Here's how the part is built. I have some questions about the finished solid (model axes, mm). A direction names the side the tool comes from. Round coordinates to 2 decimals unless told otherwise and drop trailing zeros. Order: outer loops, then holes, each group sorted by start corner. A loop starts at its lowest first (then second) coordinate and runs counter-clockwise, first axis right, second up. Notation, with made-up numbers: (-19, 78) -> (14, 78) arc R24 cw to (14, 102) -> close; hole circle Ø4 at (75, 84.5). An arc over 180 degrees is marked (long way). Answer in a Markdown table with one row per item.
```python
from build123d import *

# Parameters (mm, degrees)
SKETCH1_W           = 25
SKETCH1_H           = 50
SKETCH1_R           = 3.4
BOSS_EXTRUDE1_DEPTH = 3
SKETCH2_W           = 50
SKETCH2_H           = 3
BOSS_EXTRUDE2_DEPTH = 8
SKETCH3_W           = 8
SKETCH3_H           = 50
BOSS_EXTRUDE3_DEPTH = 42
SKETCH4_R           = 2.65
CUT_EXTRUDE1_DEPTH  = 0.5
SKETCH5_R           = 5.802370205
CUT_EXTRUDE2_DEPTH  = 9
FILLET2_R           = 1
SKETCH6_R           = 12.6
BOSS_EXTRUDE4_DEPTH = 2
FILLET4_R           = 1
SKETCH8_R           = 1.589780168
SKETCH8_R_2         = 1.777428262
CUT_EXTRUDE3_DEPTH  = 10
SKETCH9_W           = 49.021678163
SKETCH9_H           = 20.976854622
CUT_EXTRUDE4_DEPTH  = 68.79439129
SKETCH11_R          = 2.1
CUT_EXTRUDE5_DEPTH  = 59.480168703
SKETCH14_R          = 2.6
CUT_EXTRUDE6_DEPTH  = 0.5


with BuildPart() as part:
    # Sketch1 → Boss-Extrude1 (new body)
    with BuildSketch(Plane(origin=(0, 0, 0), x_dir=(1, 0, 0), z_dir=(0, 1, 0))):
        with Locations((2.276951673, 11.384758364)):
            Rectangle(SKETCH1_W, SKETCH1_H)
        with Locations(Location((1.276951673, 11.384758364, 0), (0, 0, 270))):
            Circle(SKETCH1_R, mode=Mode.SUBTRACT)
    extrude(amount=BOSS_EXTRUDE1_DEPTH)

    # Sketch2 → Boss-Extrude2 (add)
    with BuildSketch(Plane.ZY.offset(10.223048327)):
        with Locations((-11.384758364, 1.5)):
            Rectangle(SKETCH2_W, SKETCH2_H)
    extrude(amount=BOSS_EXTRUDE2_DEPTH)

    # Sketch3 → Boss-Extrude3 (add)
    with BuildSketch(Plane.XZ):
        with Locations((-14.223048327, -11.384758364)):
            Rectangle(SKETCH3_W, SKETCH3_H)
    extrude(amount=BOSS_EXTRUDE3_DEPTH)

    # Sketch4 → Cut-Extrude1 (cut)
    with BuildSketch(Plane(origin=(0, 3, 0), x_dir=(1, 0, 0), z_dir=(0, 1, 0))):
        with Locations(Location((-14.223048327, 32.384758364, 0), (0, 0, 270))):
            Circle(SKETCH4_R)
        with Locations(Location((-14.223048327, -9.615241636, 0), (0, 0, 270))):
            Circle(SKETCH4_R)
    cut_extrude1 = extrude(amount=-CUT_EXTRUDE1_DEPTH, mode=Mode.SUBTRACT)

    # Mirror1: Cut-Extrude1 across plane
    add(cut_extrude1.mirror(Plane.ZX.offset(-19.5)), mode=Mode.SUBTRACT)

    # Sketch5 → Cut-Extrude2 (cut)
    with BuildSketch(Plane.ZY.offset(18.223048327)):
        with Locations((-11.836279124, -21)):
            Circle(SKETCH5_R)
    extrude(amount=-CUT_EXTRUDE2_DEPTH, mode=Mode.SUBTRACT)

    # Fillet2
    fillet2_edges = [part.edges().sort_by_distance(p)[0] for p in [
        (-10.223048327, -21, -17.638649329),
    ]]
    fillet(fillet2_edges, radius=FILLET2_R)

    # Mirror2: Cut-Extrude1 across plane
    add(cut_extrude1.mirror(Plane.ZY.offset(1.723048327)), mode=Mode.SUBTRACT)

    # Sketch6 → Boss-Extrude4 (add)
    with BuildSketch(Plane(origin=(0, 3, 0), x_dir=(1, 0, 0), z_dir=(0, 1, 0))):
        with BuildLine():
            Line((14.776951673, 5.825082115), (14.776951673, 16.944434614))
            ThreePointArc((14.776951673, 16.944434614), (-13.323048327, 11.384758364), (14.776951673, 5.825082115))
        make_face()
        with Locations(Location((1.276951673, 11.384758364, 0), (0, 0, 270))):
            Circle(SKETCH6_R, mode=Mode.SUBTRACT)
    extrude(amount=BOSS_EXTRUDE4_DEPTH)

    # Fillet4
    # the kernel refuses this fillet: 1 mm, written as the material it takes off along each edge
    with BuildSketch(Plane(origin=(14.776951673, 5, -3.325082115), x_dir=(0, -1, 0), z_dir=(0, 0, -1))) as fillet4_piece_1:
        with BuildLine():
            CenterArc((FILLET4_R, FILLET4_R), FILLET4_R, 180, 90)
            Line((0, FILLET4_R), (0, 0))
            Line((0, 0), (FILLET4_R, 0))
        make_face()
    extrude(amount=16.119352499, mode=Mode.SUBTRACT)

    # Sketch8 → Cut-Extrude3 (cut)
    with BuildSketch(Plane(origin=(0, 3, 0), x_dir=(1, 0, 0), z_dir=(0, 1, 0))):
        with Locations(Location((1.276951673, 19.884758364, 0), (0, 0, 270))):
            Circle(SKETCH8_R)
        with Locations(Location((1.276951673, 2.884758364, 0), (0, 0, 270))):
            Circle(SKETCH8_R_2)
    extrude(amount=-CUT_EXTRUDE3_DEPTH, mode=Mode.SUBTRACT)

    # Sketch9 → Cut-Extrude4 (cut, through all)
    with BuildSketch(Plane.XY.offset(13.615241636)):
        with Locations((-9.733887409, 10.488427311)):
            Rectangle(SKETCH9_W, SKETCH9_H)
    extrude(amount=-CUT_EXTRUDE4_DEPTH, mode=Mode.SUBTRACT)

    # Sketch11 → Cut-Extrude5 (cut, through all)
    with BuildSketch(Plane(origin=(0, 0, 0), x_dir=(1, 0, 0), z_dir=(0, 1, 0))):
        with Locations(Location((-14.223048327, 32.384758364, 0), (0, 0, 270))):
            Circle(SKETCH11_R)
    cut_extrude5 = extrude(amount=-CUT_EXTRUDE5_DEPTH, mode=Mode.SUBTRACT)

    # Mirror3: Cut-Extrude5 across plane
    add(cut_extrude5.mirror(Plane.XY.offset(-11.384758364)), mode=Mode.SUBTRACT)

    # Sketch14 → Cut-Extrude6 (cut)
    with BuildSketch(Plane(origin=(0, 0, 0), x_dir=(1, 0, 0), z_dir=(0, 1, 0))):
        with Locations(Location((-14.223048327, -9.615241636, 0), (0, 0, 270))):
            Circle(SKETCH14_R)
    cut_extrude6 = extrude(amount=-CUT_EXTRUDE6_DEPTH, mode=Mode.SUBTRACT)

    # Mirror4: Cut-Extrude6 across plane
    add(cut_extrude6.mirror(Plane.XY.offset(-11.384758364)), mode=Mode.SUBTRACT)


solid = part.part
```
1. Suppose I cut it at D-D on z = 8.5. Write out the boundary of the cut face in (x, y), then the cut area to 3 significant figures.
Numbers:
| item | result |
|---|---|
| outline | (-18.22, -42) -> (-16.63, -42) -> (-16.63, -41.5) -> (-16, -41.5) -> (-16, -0.5) -> (-16.57, -0.5) -> (-16.57, 0) -> (-18.22, 0) -> close; (-12.44, -41.5) -> (-11.82, -41.5) -> (-11.82, -42) -> (-10.22, -42) -> (-10.22, 0) -> (-11.87, 0) -> (-11.87, -0.5) -> (-12.44, -0.5) -> close |
| area | 185 mm2 |
2. We'd pull the mould along Z, two halves only. Please class faces 4 (the face through (-16.76, -0.25, -31.82)), 5 (the face through (-14, -21, -36.385)), 6 (the face through (-14, -42, -11)): released by +Z, released by -Z, zero draft, split by the parting line, or undercut.
Numbers:
| item | result |
|---|---|
| face 4 | undercut |
| face 5 | released by -Z |
| face 6 | zero draft |
3. Please list where these lines run through material, in increasing order: line 1 along Z through (x, y) = (-14, -14); line 2 along Y through (x, z) = (-12.5, -12); line 3 along Z through (x, y) = (-13.5, -36).
Numbers:
| item | result |
|---|---|
| line 1 | z = -36.38 to -34.47, -30.3 to 7.53, 11.7 to 13.62 |
| line 2 | y = -42 to -26.8, -15.2 to 0 |
| line 3 | z = -36.38 to -34.36, -30.41 to 7.64, 11.59 to 13.62 |
4. For faces 1 (the face through (-11.596, -41.754, 9.27)), 2 (the face through (-16.273, -20.713, -32.84)), 3 (the face through (-16.76, -0.25, 9.05)), which set-ups out of +Z, -Z, +X, -X, +Y, -Y let a thin tool reach every point of the face, with its end or its side?
Numbers:
| item | result |
|---|---|
| face 1 | -Y |
| face 2 | +Y, -Y |
| face 3 | +Y |
5. Suppose I cut it at A-A on z = -32.5. Write out the boundary of the cut face in (x, y).
Numbers:
| item | result |
|---|---|
| outline | (-18.22, -42) -> (-16.87, -42) -> (-16.87, -41.5) -> (-16.32, -41.5) -> (-16.32, -0.5) -> (-16.82, -0.5) -> (-16.82, 0) -> (-18.22, 0) -> close; (-12.13, -41.5) -> (-11.58, -41.5) -> (-11.58, -42) -> (-10.22, -42) -> (-10.22, 0) -> (-11.63, 0) -> (-11.63, -0.5) -> (-12.13, -0.5) -> close |
6. Suppose I cut it at C-C on y = -36. Write out the boundary of the cut face in (x, z).
Numbers:
| item | result |
|---|---|
| outline | (-18.22, -36.38) -> (-10.22, -36.38) -> (-10.22, 13.62) -> (-18.22, 13.62) -> close; hole circle Ø4.2 at (-14.22, -32.38); hole circle Ø4.2 at (-14.22, 9.62) |
7. For pin 1 Ø4 at (x, z) = (-14.5, 10.5) entering from +Y, with a flat end and sliding along its axis, tell me the tip position at first contact or that it passes through.
Numbers:
| item | result |
|---|---|
| pin 1 | stops at y = 0 |
8. Suppose I cut it at B-B on y = -21. Write out the boundary of the cut face in (x, z).
Numbers:
| item | result |
|---|---|
| outline | (-18.22, -36.38) -> (-10.22, -36.38) -> (-10.22, -18.64) arc R1 ccw to (-11.22, -17.64) -> (-18.22, -17.64) -> close; (-18.22, -6.03) -> (-11.22, -6.03) arc R1 ccw to (-10.22, -5.03) -> (-10.22, 13.62) -> (-18.22, 13.62) -> close; hole circle Ø4.2 at (-14.22, -32.38); hole circle Ø4.2 at (-14.22, 9.62) |
